For this review, take the finished solid that the model builds, in its own axes (mm). Face numbers are marked on the shaded views. A direction names the side the tool comes from. Give positions to 0.01 mm unless a question says otherwise; leave off trailing zeros. Order: outer loops, then holes, each group sorted by start corner. A loop starts at its lowest first (then second) coordinate and runs counter-clockwise, first axis right, second up. Notation, with made-up numbers: (74.25, -39.75) -> (122.25, -39.75) arc R37 cw to (122.25, -2.75) -> close; hole circle Ø2 at (37, 49). An arc over 180 degrees is marked (long way). Return JSON: item names as keys, results as strings. Group by question number.
1) Add section A-A (y = -55). Give the boundary of the cut face in (x, z).
2) For the marked faces 1, 2, 3, 4 and 5, list the 3-axis set-ups (+Z, -Z, +X, -X, +Y, -Y) from which the entire face can be reached by the end or side of a thin tool; tool diameter is ignored.
3) Add section C-C (z = 24). Give the boundary of the cut face in (x, y).
4) Add section D-D (y = -35.5). Give the boundary of the cut face in (x, z), then the cut area to 3 significant figures.
5) To check wall thickness, follow line 1 along Y through (x, z) = (-41.5, 6); line 2 along X through (y, z) = (37, 8); line 3 along X through (y, z) = (-54.5, 20.5). State the ranges of each line that lie inside material, in increasing order.
6) The part is to be moulded in two halves that separate along X. For the marked faces 6, 7, 8 and 9, say which applies: released by +X, released by -X, zero draft, split by the parting line, or undercut.
7) Insertion check: P1, Ø8, axis at x = 42.5, z = 21, coming from the +Y side; P2, Ø12, axis at y = 43, z = 32.5, coming from the +X side; P3, Ø8, axis at y = -20.5, z = 5, coming from the +X side; P4, Ø9, axis at x = -55, y = 0, coming from the -Z side. Each pin has a flat end and moves straight along its axis. Give the tip position at first contact, or say it passes through.
from build123d import *

# Parameters (mm, degrees)
SKETCH2_R           = 5
SKETCH2_R_2         = 40
BOSS_EXTRUDE1_DEPTH = 30
SKETCH2_4_R         = 40
SKETCH2_4_R_2       = 30
BOSS_EXTRUDE2_DEPTH = 40
SKETCH2_5_R         = 30
BOSS_EXTRUDE3_DEPTH = 10
SKETCH3_W           = 75
SKETCH3_H           = 75
CUT_EXTRUDE1_DEPTH  = 40


with BuildPart() as part:
    # Sketch2 → Boss-Extrude1 (new body)
    with BuildSketch(Plane.XY):
        with BuildLine():
            ThreePointArc((-62.292670356, 9.529793233), (-52.807960272, 21.873773346), (-50.786151046, 37.308988209))
            ThreePointArc((-50.786151046, 37.308988209), (-47.376154339, 47.376154339), (-37.308988209, 50.786151046))
            ThreePointArc((-37.308988209, 50.786151046), (-21.873773346, 52.807960272), (-9.529793233, 62.292670356))
            ThreePointArc((-9.529793233, 62.292670356), (0, 67), (9.529793233, 62.292670356))
            ThreePointArc((9.529793233, 62.292670356), (21.873773346, 52.807960272), (37.308988209, 50.786151046))
            ThreePointArc((37.308988209, 50.786151046), (47.376154339, 47.376154339), (50.786151046, 37.308988209))
            ThreePointArc((50.786151046, 37.308988209), (52.807960272, 21.873773346), (62.292670356, 9.529793233))
            ThreePointArc((62.292670356, 9.529793233), (67, 0), (62.292670356, -9.529793233))
            ThreePointArc((62.292670356, -9.529793233), (52.807960272, -21.873773346), (50.786151046, -37.308988209))
            ThreePointArc((50.786151046, -37.308988209), (47.376154339, -47.376154339), (37.308988209, -50.786151046))
            ThreePointArc((37.308988209, -50.786151046), (21.873773346, -52.807960272), (9.529793233, -62.292670356))
            ThreePointArc((9.529793233, -62.292670356), (0, -67), (-9.529793233, -62.292670356))
            ThreePointArc((-9.529793233, -62.292670356), (-21.873773346, -52.807960272), (-37.308988209, -50.786151046))
            ThreePointArc((-37.308988209, -50.786151046), (-47.376154339, -47.376154339), (-50.786151046, -37.308988209))
            ThreePointArc((-50.786151046, -37.308988209), (-52.807960272, -21.873773346), (-62.292670356, -9.529793233))
            ThreePointArc((-62.292670356, -9.529793233), (-67, 0), (-62.292670356, 9.529793233))
        make_face()
        with Locations((-38.890872965, -38.890872965)):
            Circle(SKETCH2_R, mode=Mode.SUBTRACT)
        with Locations((0, -55)):
            Circle(SKETCH2_R, mode=Mode.SUBTRACT)
        with Locations((38.890872965, -38.890872965)):
            Circle(SKETCH2_R, mode=Mode.SUBTRACT)
        with Locations((55, 0)):
            Circle(SKETCH2_R, mode=Mode.SUBTRACT)
        with Locations((38.890872965, 38.890872965)):
            Circle(SKETCH2_R, mode=Mode.SUBTRACT)
        with Locations((0, 55)):
            Circle(SKETCH2_R, mode=Mode.SUBTRACT)
        with Locations((-38.890872965, 38.890872965)):
            Circle(SKETCH2_R, mode=Mode.SUBTRACT)
        with Locations((-55, 0)):
            Circle(SKETCH2_R, mode=Mode.SUBTRACT)
        Circle(SKETCH2_R_2, mode=Mode.SUBTRACT)
    extrude(amount=BOSS_EXTRUDE1_DEPTH)

    # Sketch2_4 → Boss-Extrude2 (add)
    with BuildSketch(Plane.XY):
        Circle(SKETCH2_4_R)
        Circle(SKETCH2_4_R_2, mode=Mode.SUBTRACT)
    extrude(amount=BOSS_EXTRUDE2_DEPTH)

    # Sketch2_5 → Boss-Extrude3 (add)
    with BuildSketch(Plane.XY):
        Circle(SKETCH2_5_R)
        with BuildLine():
            ThreePointArc((-14.696938457, -3), (-10.606601718, -10.606601718), (-3, -14.696938457))
            Line((-3, -14.696938457), (-3, -24.819347292))
            ThreePointArc((-3, -24.819347292), (0, -25), (3, -24.819347292))
            Line((3, -24.819347292), (3, -14.696938457))
            ThreePointArc((3, -14.696938457), (10.606601718, -10.606601718), (14.696938457, -3))
            Line((14.696938457, -3), (24.819347292, -3))
            ThreePointArc((24.819347292, -3), (25, 0), (24.819347292, 3))
            Line((24.819347292, 3), (14.696938457, 3))
            ThreePointArc((14.696938457, 3), (10.606601718, 10.606601718), (3, 14.696938457))
            Line((3, 14.696938457), (3, 24.819347292))
            ThreePointArc((3, 24.819347292), (0, 25), (-3, 24.819347292))
            Line((-3, 24.819347292), (-3, 14.696938457))
            ThreePointArc((-3, 14.696938457), (-10.606601718, 10.606601718), (-14.696938457, 3))
            Line((-14.696938457, 3), (-24.819347292, 3))
            ThreePointArc((-24.819347292, 3), (-25, 0), (-24.819347292, -3))
            Line((-24.819347292, -3), (-14.696938457, -3))
        make_face(mode=Mode.SUBTRACT)
    extrude(amount=BOSS_EXTRUDE3_DEPTH)

    # Sketch3 → Cut-Extrude1 (cut)
    with BuildSketch(Plane.XY):
        with Locations((37.5, 37.5)):
            Rectangle(SKETCH3_W, SKETCH3_H)
    extrude(amount=CUT_EXTRUDE1_DEPTH, mode=Mode.SUBTRACT)


solid = part.part
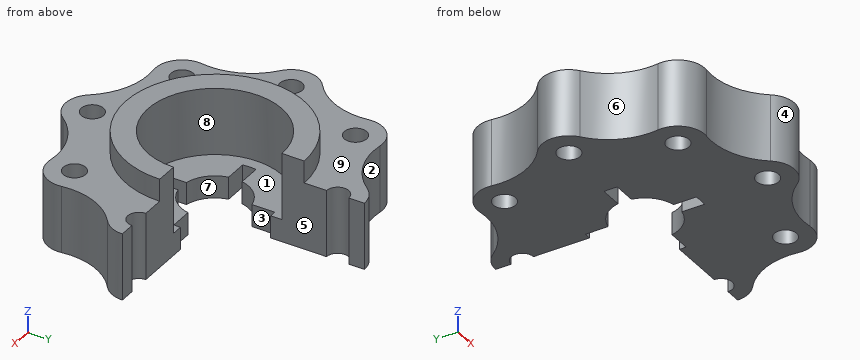
Evaluation:
{
 "1": {"outline": "(-17.59, 0) -> (-5, 0) -> (-5, 30) -> (-17.59, 30) -> close; (5, 0) -> (17.59, 0) -> (17.59, 30) -> (5, 30) -> close"},
 "2": {"face 1": "+Z", "face 2": "+Z, -Z, +Y", "face 3": "+Z, -Z, +X", "face 4": "+Z, -Z, -Y", "face 5": "+Z, -Z, +X, +Y"},
 "3": {"outline": "(-62.29, -9.53) arc R30 cw to (-50.79, -37.31) arc R12 ccw to (-37.31, -50.79) arc R30 cw to (-9.53, -62.29) arc R12 ccw to (9.53, -62.29) arc R30 cw to (37.31, -50.79) arc R12 ccw to (50.79, -37.31) arc R30 cw to (62.29, -9.53) arc R12 ccw to (67, 0) -> (60, 0) arc R5 cw to (50, 0) -> (30, 0) arc R30 cw (long way) to (0, 30) -> (0, 50) arc R5 cw to (0, 60) -> (0, 67) arc R12 ccw to (-9.53, 62.29) arc R30 cw to (-37.31, 50.79) arc R12 ccw to (-50.79, 37.31) arc R30 cw to (-62.29, 9.53) arc R12 ccw to start; hole circle Ø10 at (-55, 0); hole circle Ø10 at (-38.89, -38.89); hole circle Ø10 at (-38.89, 38.89); hole circle Ø10 at (0, -55); hole circle Ø10 at (38.89, -38.89)"},
 "4": {"outline": "(-50.6, 0) -> (-42.57, 0) -> (-42.57, 30) -> (-50.6, 30) -> close; (-35.22, 0) -> (35.22, 0) -> (35.22, 30) -> (18.43, 30) -> (18.43, 40) -> (-18.43, 40) -> (-18.43, 30) -> (-35.22, 30) -> close; (42.57, 0) -> (50.6, 0) -> (50.6, 30) -> (42.57, 30) -> close", "area": "2,960 mm^2"},
 "5": {"line 1": "-50.6 to -43.16, -34.63 to 34.63, 43.16 to 50.6", "line 2": "-50.75 to -43.52, -34.26 to 0", "line 3": "-18.43 to -4.97, 4.97 to 18.43"},
 "6": {"face 6": "released by -X", "face 7": "undercut", "face 8": "undercut", "face 9": "zero draft"},
 "7": {"P1": "y = 0", "P2": "x = 0", "P3": "x = 55.71", "P4": "through"}
}
